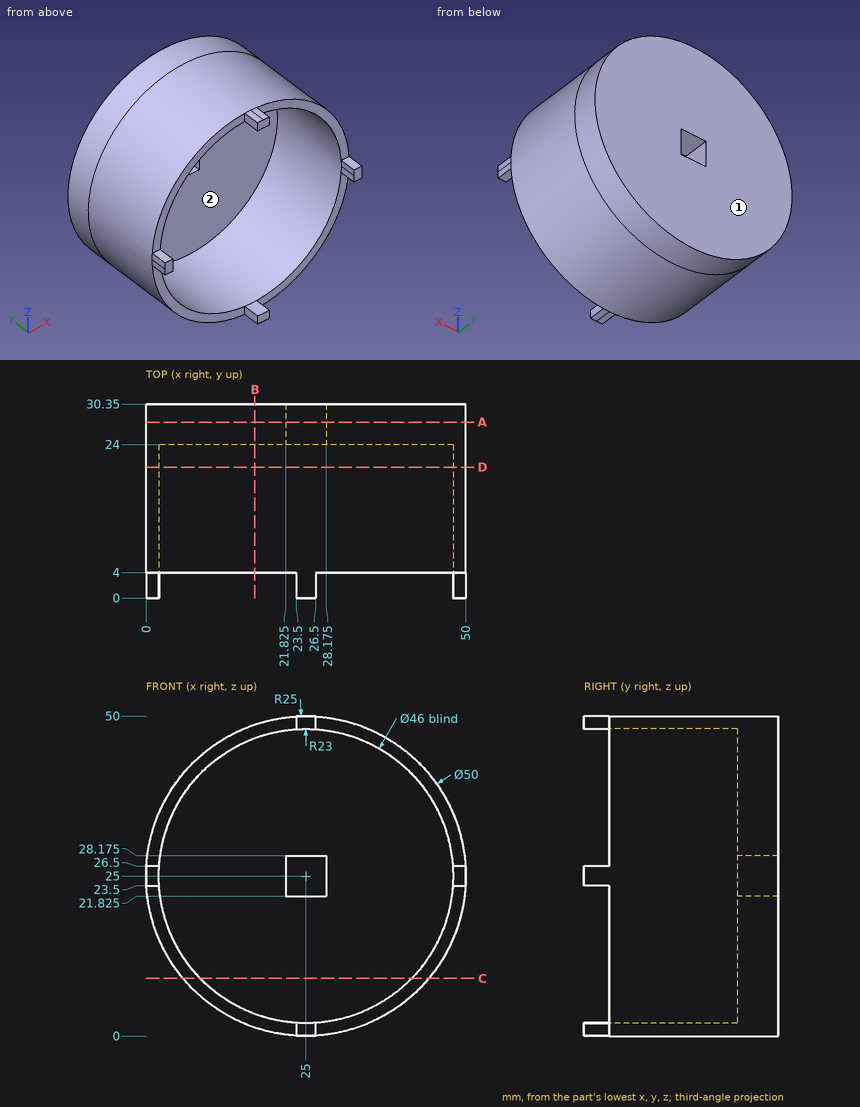
Design review of the part shown in the three views and the two pictorial views. Dimensions are in mm from the part's minimum x, y and z. Round coordinates to 2 decimals unless told otherwise and drop trailing zeros. Loops run counter-clockwise (first coordinate to the right, second up) from the corner with the lowest first, then second, coordinate; pieces in that order, holes last. Notation, with made-up numbers: (76.5, 61) - (130.5, 61) arc R16 cw to (130.5, 70) - close; hole circle Ø11 at (12.5, 28). An arc over 180 degrees is marked (long way). Use CSV: the item, a comma, the result in double quotes.
(1) Take a section at D-D, the plane y = 20.5. Give the boundary of the cut face in (x, z), plus the area to 3 significant figures.
Working result:
outline,"circle Ø50 at (25, 25); hole circle Ø46 at (25, 25)"
area,"302 mm^2"
(2) Take a section at B-B, the plane x = 17. Give the boundary of the cut face in (y, z), plus the area to 3 significant figures.
Working result:
outline,"(4, 1.31) - (30.35, 1.31) - (30.35, 48.69) - (4, 48.69) - (4, 46.56) - (24, 46.56) - (24, 3.44) - (4, 3.44) - close"
area,"386 mm^2"
(3) The part is to be moulded in two halves that separate along X. For the marked faces 1 and 2, say which applies: pulls with the +X half, pulls with the -X half, needs draft (parallel to the pull), parting line crosses it, or undercut.
Working result:
face 1,"needs draft"
face 2,"undercut"
(4) For line 1 (X direction, y = 13, z = 25); line 2 (Y direction, x = 39, z = 10), list the stretches that pass through material, from the lowest coordinate up.
Working result:
line 1,"x = 0 to 2, 48 to 50"
line 2,"y = 24 to 30.35"
(5) Take a section at A-A, the plane y = 27.5. Give the boundary of the cut face in (x, z) (3 decimals).
Working result:
outline,"circle Ø50 at (25, 25); hole (21.825, 21.825) - (28.175, 21.825) - (28.175, 28.175) - (21.825, 28.175) - close"
(6) Take a section at C-C, the plane z = 9. Give the boundary of the cut face in (x, y).
Working result:
outline,"(5.79, 4) - (8.48, 4) - (8.48, 24) - (41.52, 24) - (41.52, 4) - (44.21, 4) - (44.21, 30.35) - (5.79, 30.35) - close"
(7) Clearance check with flat-ended pins moving along their axes: P1, Ø12, axis at x = 10.5, y = 22, coming from the +Z side; P2, Ø1.6, axis at x = 0.5, y = 1.5, coming from the +Z side; P3, Ø5, axis at x = 11.5, z = 16.5, coming from the -Y side. State where each tip first meets the part, or that it passes through.
Working result:
P1,"stops at z = 48.51"
P2,"stops at z = 26.5"
P3,"stops at y = 24"
